Can you work these out from the model? Positions are in its coordinate system, mm. A direction names the side the tool comes from. Give positions to 0.01 mm unless a question says otherwise; leave off trailing zeros.
```python
from build123d import *

# Parameters (mm, degrees)
SKIZZE2_W                        = 120
SKIZZE2_H                        = 39.364160046
AUFSATZ_LINEAR_AUSTRAGEN1_DEPTH  = 30
SKIZZE24_R                       = 1.55
SCHNITT_LINEAR_AUSTRAGEN4_DEPTH  = 130.805766806
SKIZZE46_R                       = 2.85
SCHNITT_LINEAR_AUSTRAGEN15_DEPTH = 10
SCHNITT_LINEAR_START             = -5
SCHNITT_LINEAR_AUSTRAGEN25_DEPTH = 2.7
LINEARES_MUSTER1_COUNT           = 4
LINEARES_MUSTER1_PITCH           = 20
SPIEGELN2_COPY_1_SKETCH_R        = 2.85
SPIEGELN2_COPY_1_DEPTH           = 10
SPIEGELN2_COPY_2_SKETCH_R        = 2.85
SPIEGELN2_COPY_2_DEPTH           = 10
SPIEGELN2_COPY_3_SKETCH_R        = 2.85
SPIEGELN2_COPY_3_DEPTH           = 10
SPIEGELN2_START                  = -5
SPIEGELN2_COPY_4_DEPTH           = 2.7
SPIEGELN2_COPY_5_DEPTH           = 2.7
SPIEGELN2_COPY_6_DEPTH           = 2.7
SKIZZE51_R                       = 1.55
SCHNITT_LINEAR_AUSTRAGEN26_DEPTH = 130.805766806
SKIZZE75_R                       = 0.75
SCHNITT_LINEAR_AUSTRAGEN28_DEPTH = 12
SKIZZE76_R                       = 2
SCHNITT_LINEAR_AUSTRAGEN29_DEPTH = 6
SKIZZE80_R                       = 0.5
SCHNITT_LINEAR_AUSTRAGEN34_DEPTH = 21.05
SCHNITT_LINEAR_START_2           = -7.5
SKIZZE81_R                       = 0.5
SCHNITT_LINEAR_AUSTRAGEN36_DEPTH = 5
FASE1_SIZE                       = 1
ABSPALTEN3_START                 = 15
ABSPALTEN3_OUTLINE_W             = 120
ABSPALTEN3_OUTLINE_H             = 39.364160046
ABSPALTEN3_OUTLINE_R             = 1.55
ABSPALTEN3_OUTLINE_R_2           = 0.75
ABSPALTEN3_DEPTH                 = 15


# Read off the part's stored shape, not the designer's step: Abspalten3
with BuildPart() as part:
    # Skizze2 → Aufsatz-Linear austragen1 (new body)
    with BuildSketch(Plane.XY):
        with Locations((60, 19.682080023)):
            Rectangle(SKIZZE2_W, SKIZZE2_H)
    extrude(amount=AUFSATZ_LINEAR_AUSTRAGEN1_DEPTH)

    # Skizze24 → Schnitt-Linear austragen4 (cut, through all)
    with BuildSketch(Plane.XY.offset(30)):
        with Locations((40, 31.364160046)):
            Circle(SKIZZE24_R)
        with Locations((60, 31.364160046)):
            Circle(SKIZZE24_R)
        with Locations((80, 31.364160046)):
            Circle(SKIZZE24_R)
        with Locations((100, 31.364160046)):
            Circle(SKIZZE24_R)
    schnitt_linear_austragen4 = extrude(amount=-SCHNITT_LINEAR_AUSTRAGEN4_DEPTH, mode=Mode.SUBTRACT)

    # Skizze46 → Schnitt-Linear austragen15 (cut)
    with BuildSketch(Plane(origin=(0, 0, 0), x_dir=(-1, 0, 0), z_dir=(0, 0, -1))):
        with Locations((-100, 31.364160046)):
            Circle(SKIZZE46_R)
    schnitt_linear_austragen15 = extrude(amount=-SCHNITT_LINEAR_AUSTRAGEN15_DEPTH, mode=Mode.SUBTRACT)

    # Skizze50 → Schnitt-Linear austragen25 (cut)
    with BuildSketch(Plane.XY.offset(30).offset(SCHNITT_LINEAR_START)):
        Polygon((97.15, 33.009608314), (97.15, 39.364160046), (102.85, 39.364160046), (102.85, 33.009608314), (102.85, 29.718711779), (100, 28.073263512), (97.15, 29.718711779), align=None)
    schnitt_linear_austragen25 = extrude(amount=-SCHNITT_LINEAR_AUSTRAGEN25_DEPTH, mode=Mode.SUBTRACT)

    # Lineares Muster1: Schnitt-Linear austragen15, Schnitt-Linear austragen25 ×4
    with Locations(*[(-i * LINEARES_MUSTER1_PITCH, 0, 0) for i in range(1, LINEARES_MUSTER1_COUNT)]):
        add(schnitt_linear_austragen15, mode=Mode.SUBTRACT)
        add(schnitt_linear_austragen25, mode=Mode.SUBTRACT)

    # Spiegeln2: Schnitt-Linear austragen15, Schnitt-Linear austragen25 across plane
    add(schnitt_linear_austragen15.mirror(Plane.ZX.offset(19.764160046)), mode=Mode.SUBTRACT)
    add(schnitt_linear_austragen25.mirror(Plane.ZX.offset(19.764160046)), mode=Mode.SUBTRACT)

    # Spiegeln2 copy 1 sketch → Spiegeln2 copy 1 (cut)
    with BuildSketch(Plane(origin=(-20, 39.528320093, 0), x_dir=(-1, 0, 0), z_dir=(0, 0, -1))):
        with Locations((-100, -31.364160046)):
            Circle(SPIEGELN2_COPY_1_SKETCH_R)
    extrude(amount=-SPIEGELN2_COPY_1_DEPTH, mode=Mode.SUBTRACT)

    # Spiegeln2 copy 2 sketch → Spiegeln2 copy 2 (cut)
    with BuildSketch(Plane(origin=(-40, 39.528320093, 0), x_dir=(-1, 0, 0), z_dir=(0, 0, -1))):
        with Locations((-100, -31.364160046)):
            Circle(SPIEGELN2_COPY_2_SKETCH_R)
    extrude(amount=-SPIEGELN2_COPY_2_DEPTH, mode=Mode.SUBTRACT)

    # Spiegeln2 copy 3 sketch → Spiegeln2 copy 3 (cut)
    with BuildSketch(Plane(origin=(-60, 39.528320093, 0), x_dir=(-1, 0, 0), z_dir=(0, 0, -1))):
        with Locations((-100, -31.364160046)):
            Circle(SPIEGELN2_COPY_3_SKETCH_R)
    extrude(amount=-SPIEGELN2_COPY_3_DEPTH, mode=Mode.SUBTRACT)

    # Spiegeln2 copy 4 sketch → Spiegeln2 copy 4 (cut)
    with BuildSketch(Plane(origin=(-20, 39.528320093, 30), x_dir=(1, 0, 0), z_dir=(0, 0, 1)).offset(SPIEGELN2_START)):
        Polygon((97.15, -33.009608314), (97.15, -39.364160046), (102.85, -39.364160046), (102.85, -33.009608314), (102.85, -29.718711779), (100, -28.073263512), (97.15, -29.718711779), align=None)
    extrude(amount=-SPIEGELN2_COPY_4_DEPTH, mode=Mode.SUBTRACT)

    # Spiegeln2 copy 5 sketch → Spiegeln2 copy 5 (cut)
    with BuildSketch(Plane(origin=(-40, 39.528320093, 30), x_dir=(1, 0, 0), z_dir=(0, 0, 1)).offset(SPIEGELN2_START)):
        Polygon((97.15, -33.009608314), (97.15, -39.364160046), (102.85, -39.364160046), (102.85, -33.009608314), (102.85, -29.718711779), (100, -28.073263512), (97.15, -29.718711779), align=None)
    extrude(amount=-SPIEGELN2_COPY_5_DEPTH, mode=Mode.SUBTRACT)

    # Spiegeln2 copy 6 sketch → Spiegeln2 copy 6 (cut)
    with BuildSketch(Plane(origin=(-60, 39.528320093, 30), x_dir=(1, 0, 0), z_dir=(0, 0, 1)).offset(SPIEGELN2_START)):
        Polygon((97.15, -33.009608314), (97.15, -39.364160046), (102.85, -39.364160046), (102.85, -33.009608314), (102.85, -29.718711779), (100, -28.073263512), (97.15, -29.718711779), align=None)
    extrude(amount=-SPIEGELN2_COPY_6_DEPTH, mode=Mode.SUBTRACT)

    # Spiegeln3: Schnitt-Linear austragen4 across plane
    add(schnitt_linear_austragen4.mirror(Plane.ZX.offset(19.764160046)), mode=Mode.SUBTRACT)

    # Skizze51 → Schnitt-Linear austragen26 (cut, through all)
    with BuildSketch(Plane.XY.offset(30)):
        with Locations((5, 34.364160046)):
            Circle(SKIZZE51_R)
        with Locations((115, 5)):
            Circle(SKIZZE51_R)
    extrude(amount=-SCHNITT_LINEAR_AUSTRAGEN26_DEPTH, mode=Mode.SUBTRACT)

    # Skizze73 → Schnitt-Rotation5 (revolve, cut)
    with BuildSketch(Plane.XY.offset(15)):
        Polygon((15, 19.764160046), (15, 23.814160046), (20, 23.814160046), (20, 24.814160046), (100, 23.232080023), (100, 22.232080023), (105, 22.232080023), (105, 19.682080023), align=None)
    revolve(axis=Axis((105, 19.682080023, 15), (-0.9999995841280241, 0.0009119998787298228, 0)), mode=Mode.SUBTRACT)

    # Skizze75 → Schnitt-Linear austragen28 (cut)
    with BuildSketch(Plane.XY.offset(30)):
        with Locations((21.598259807, 19.682080023)):
            Circle(SKIZZE75_R)
    extrude(amount=-SCHNITT_LINEAR_AUSTRAGEN28_DEPTH, mode=Mode.SUBTRACT)

    # Skizze76 → Schnitt-Linear austragen29 (cut)
    with BuildSketch(Plane.XY.offset(30)):
        with Locations((21.598259807, 19.682080023)):
            Circle(SKIZZE76_R)
    extrude(amount=-SCHNITT_LINEAR_AUSTRAGEN29_DEPTH, mode=Mode.SUBTRACT)

    # Skizze80 → Schnitt-Linear austragen34 (cut)
    with BuildSketch(Plane(origin=(120, 0, 0), x_dir=(0, 0, -1), z_dir=(1, 0, 0))):
        with Locations((-22.000416524, 19.763714623)):
            Circle(SKIZZE80_R)
    schnitt_linear_austragen34 = extrude(amount=-SCHNITT_LINEAR_AUSTRAGEN34_DEPTH, mode=Mode.SUBTRACT)

    # Skizze81 → Schnitt-Linear austragen36 (cut)
    with BuildSketch(Plane.XY.offset(30).offset(SCHNITT_LINEAR_START_2)):
        with Locations(Location((99, 19.682080023, 0), (0, 0, 7.034090001))):
            Circle(SKIZZE81_R)
    schnitt_linear_austragen36 = extrude(amount=-SCHNITT_LINEAR_AUSTRAGEN36_DEPTH, mode=Mode.SUBTRACT)

    # Spiegeln4: Schnitt-Linear austragen34, Schnitt-Linear austragen36 across plane
    add(schnitt_linear_austragen34.mirror(Plane.XY.offset(15)), mode=Mode.SUBTRACT)
    add(schnitt_linear_austragen36.mirror(Plane.XY.offset(15)), mode=Mode.SUBTRACT)

    # Fase1
    fase1_edges = [part.edges().sort_by_distance(p)[0] for p in [
        (20.848259807, 19.682080023, 24),
    ]]
    chamfer(fase1_edges, length=FASE1_SIZE)

    # Abspalten3 outline → Abspalten3 (cut)
    with BuildSketch(Plane.XY.offset(ABSPALTEN3_START)):
        with Locations((60, 19.682080023)):
            Rectangle(ABSPALTEN3_OUTLINE_W, ABSPALTEN3_OUTLINE_H)
        with Locations((115, 5)):
            Circle(ABSPALTEN3_OUTLINE_R, mode=Mode.SUBTRACT)
        with Locations((5, 34.364160046)):
            Circle(ABSPALTEN3_OUTLINE_R, mode=Mode.SUBTRACT)
        with Locations((40, 31.364160046)):
            Circle(ABSPALTEN3_OUTLINE_R, mode=Mode.SUBTRACT)
        with Locations((60, 31.364160046)):
            Circle(ABSPALTEN3_OUTLINE_R, mode=Mode.SUBTRACT)
        with Locations((80, 31.364160046)):
            Circle(ABSPALTEN3_OUTLINE_R, mode=Mode.SUBTRACT)
        with Locations((100, 31.364160046)):
            Circle(ABSPALTEN3_OUTLINE_R, mode=Mode.SUBTRACT)
        with Locations((40, 8.164160046)):
            Circle(ABSPALTEN3_OUTLINE_R, mode=Mode.SUBTRACT)
        with Locations((60, 8.164160046)):
            Circle(ABSPALTEN3_OUTLINE_R, mode=Mode.SUBTRACT)
        with Locations((80, 8.164160046)):
            Circle(ABSPALTEN3_OUTLINE_R, mode=Mode.SUBTRACT)
        with Locations((100, 8.164160046)):
            Circle(ABSPALTEN3_OUTLINE_R, mode=Mode.SUBTRACT)
        with Locations((21.598259807, 19.682080023)):
            Circle(ABSPALTEN3_OUTLINE_R_2, mode=Mode.SUBTRACT)
    extrude(amount=ABSPALTEN3_DEPTH, mode=Mode.SUBTRACT)


solid = part.part
```
1) If we mould it in two halves opening along Y, with no side actions, what happens to faces 4 (the face through (81.43, 30.77, 12.54)), 5 (the face through (59.2, 24.3, 15)), 6 (the face through (17.53, 19.85, 10.95))? For each: +Y half, -Y half, draft (parallel to the pull), parting line (faces both ways), or undercut.
Values follow:
face 4: undercut
face 5: draft
face 6: undercut
2) Suppose I cut it at A-A on z = 2. State how many separate pieces and enclosed holes the cut face has, plus the area to 3 significant figures.
Values follow:
separate pieces: 1
enclosed holes: 10
area: 4,500 mm2
3) For pin 1 Ø1.7 at (x, y) = (79.5, 9.5) entering from -Z; pin 2 Ø3 at (x, y) = (60, 31.36) entering from +Z, each with a flat end and sliding along its axis, tell me the tip position at first contact or that it passes through.
Values follow:
pin 1: stops at z = 10
pin 2: passes through
4) For faces 1 (the face through (99.998, 19.746, 12.296)), 2 (the face through (61.48, 31.83, 12.54)), 3 (the face through (78.8, 30.1, 10)), which set-ups out of +Z, -Z, +X, -X, +Y, -Y let a thin tool reach every point of the face, with its end or its side?
Values follow:
face 1: +Z
face 2: +Z, -Z
face 3: -Z
5) Please list where these lines run through material, in increasing order: L1, parallel to Y at x = 60, z = 8.25; L2, parallel to X at y = 31, z = 5.75; L3, parallel to X at y = 22.5, z = 13.5.
Values follow:
L1: y = 0 to 5.31, 11.01 to 28.51, 34.21 to 39.36
L2: x = 0 to 37.17, 42.83 to 57.17, 62.83 to 77.17, 82.83 to 97.17, 102.83 to 120
L3: x = 0 to 15, 100 to 120
